Work out the finished part from the listing and answer in its coordinate system (mm). Face numbers are marked on the shaded views. Give positions to 0.01 mm unless a question says otherwise; leave off trailing zeros. Order: outer loops, then holes, each group sorted by start corner. A loop starts at its lowest first (then second) coordinate and runs counter-clockwise, first axis right, second up. Notation, with made-up numbers: (-18, 79) - (18, 79) arc R30 ccw to (18, 115) - close; hole circle Ø6 at (45.25, 30.25). An arc over 180 degrees is marked (long way). Put each result on its own line as item: value.
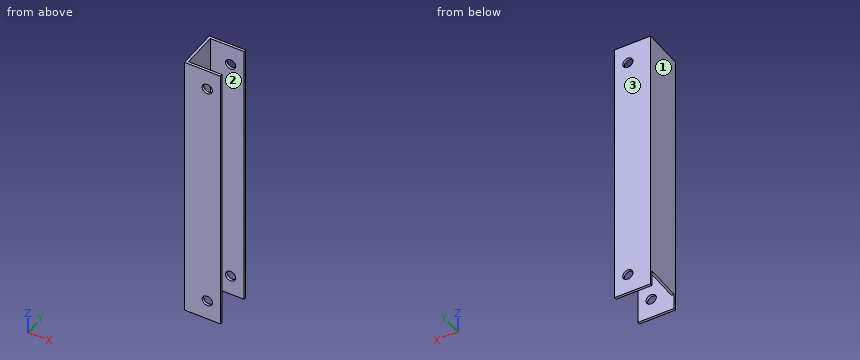
```python
from build123d import *

# Parameters (mm, degrees)
SALIENTE_EXTRUIR1_DEPTH = 175
CROQUIS2_R              = 6.5
CORTAR_EXTRUIR1_DEPTH   = 300
CROQUIS3_W              = 20
CROQUIS3_H              = 46
CORTAR_EXTRUIR2_DEPTH   = 10


with BuildPart() as part:
    # Croquis1 → Saliente-Extruir1 (new, symmetric)
    with BuildSketch(Plane.XY):
        Polygon((23, 23), (-19.825, 23), (-19.825, -23), (23, -23), (23, -26.175), (-23, -26.175), (-23, 26.175), (23, 26.175), align=None)
    extrude(amount=SALIENTE_EXTRUIR1_DEPTH, both=True)

    # Croquis2 → Cortar-Extruir1 (cut)
    with BuildSketch(Plane.XZ.offset(26.175)):
        with Locations(Location((6, 149.6, 0), (0, 0, 90))):
            Circle(CROQUIS2_R)
        with Locations(Location((6, -149.6, 0), (0, 0, 90))):
            Circle(CROQUIS2_R)
    extrude(amount=-CORTAR_EXTRUIR1_DEPTH, mode=Mode.SUBTRACT)

    # Croquis3 → Cortar-Extruir2 (cut)
    with BuildSketch(Plane.ZY.offset(23)):
        with Locations((-165, 0)):
            Rectangle(CROQUIS3_W, CROQUIS3_H)
    extrude(amount=-CORTAR_EXTRUIR2_DEPTH, mode=Mode.SUBTRACT)


solid = part.part
```
(1) Section A-A, the plane x = 16.5 is taken. Write down the section's boundary in (y, z) (3 decimals), then the cut area to 3 significant figures.
Geometry check:
outline: (-26.175, -175) - (-23, -175) - (-23, 175) - (-26.175, 175) - close; (23, -175) - (26.175, -175) - (26.175, 175) - (23, 175) - close
area: 2,220 mm²
(2) Straight lines are drawn through the part: line 1 (Y direction, x = 8, z = -98) (3 decimals); line 2 (X direction, y = 24, z = 149); line 3 (X direction, y = 9, z = -146) (3 decimals). For each, find the intervals that lie inside material, in ascending order.
Geometry check:
line 1: y = -26.175 to -23, 23 to 26.175
line 2: x = -23 to -0.47, 12.47 to 23
line 3: x = -23 to -19.825
(3) Section D-D, the plane z = 38 is taken. Write down the section's boundary in (x, y) (3 decimals), then the cut area to 3 significant figures.
Geometry check:
outline: (-23, -26.175) - (23, -26.175) - (23, -23) - (-19.825, -23) - (-19.825, 23) - (23, 23) - (23, 26.175) - (-23, 26.175) - close
area: 438 mm²
(4) Determine the mould class of the marked faces 1, 2 and 3 for opening direction Y: pulls with the +Y half, pulls with the -Y half, needs draft (parallel to the pull), parting line crosses it, or undercut.
Geometry check:
face 1: needs draft
face 2: undercut
face 3: pulls with the +Y half
(5) Given pin 1 (1.5 mm diameter, centred on y = 0, z = 91, fed in from +X) (3 decimals); pin 2 (21 mm diameter, centred on x = 6, z = 149.6, fed in from -Y) (3 decimals); pin 3 (2.5 mm diameter, centred on x = -21.5, y = 0, fed in from -Z), each flat-ended and moving along its own axis, determine where each tip first touches the part or whether it passes through.
Geometry check:
pin 1: stops at x = -19.825
pin 2: stops at y = -26.175
pin 3: stops at z = -155
(6) Section B-B, the plane z = -149.6 is taken. Write down the section's boundary in (x, y) (3 decimals), then the cut area to 3 significant figures.
Geometry check:
outline: (-23, -26.175) - (-0.5, -26.175) - (-0.5, -23) - (-19.825, -23) - (-19.825, 23) - (-0.5, 23) - (-0.5, 26.175) - (-23, 26.175) - close; (12.5, -26.175) - (23, -26.175) - (23, -23) - (12.5, -23) - close; (12.5, 23) - (23, 23) - (23, 26.175) - (12.5, 26.175) - close
area: 356 mm²
(7) Section C-C, the plane y = 8.5 is taken. Write down the section's boundary in (x, z) (3 decimals).
Geometry check:
outline: (-23, -155) - (-19.825, -155) - (-19.825, 175) - (-23, 175) - close
